Autodesk Inventor part; units mm, degrees
ref_plane "YZ Plane" through (0, 0, 0) normal (1, 0, 0) x (0, 1, 0)
ref_plane "XZ Plane" through (0, 0, 0) normal (0, 1, 0) x (-1, 0, 0)
ref_plane "XY Plane" through (0, 0, 0) normal (0, 0, 1) x (1, 0, 0)
sketch "Sketch1" plane through (0, 0, 0) normal (0, 0, 1) x (1, 0, 0)
  circle A0 centre (10, 11.5) radius 1.6
  line L0 (0, 0) -> (20.0001, 0)
  line L1 (0, 0) -> (0, 3)
  line L2 (20.0001, 0) -> (20.0001, 3)
  line L3 (0, 3) -> (16, 3) construction
  line L4 (20.0001, 3) -> (36.0001, 3) construction
  arc A1 (14.3301, 14) -> (5.6699, 14) centre (10, 11.5) ccw
  line L5 (10, 11.5) -> (5.6699, 14) construction
  line L6 (10, 11.5) -> (14.3301, 14) construction
  line L7 (5.6699, 14) -> (0, 3)
  line L8 (14.3301, 14) -> (20.0001, 3)
  dimension "d17" = 3
  dimension "d18" = 3
  dimension "d19" = 11.5
  dimension "d23" = 90
  dimension "d24" = 90
  dimension "d25" = 10
  dimension "d31" = 5
  dimension "d32" = 120
  dimension "d33" = 14
extrude "Extrusion1" add sketch "Sketch1" along normal blind 4.5
sketch "Sketch4" plane through (0, 0, 4.5) normal (0, 0, 1) x (1, 0, 0)
  line L0 (0, 3) -> (0, 0)
  line L1 (20.0001, 0) -> (20.0001, 3)
  line L2 (0, 0) -> (20.0001, 0)
  line L3 (20.0001, 0) -> (20.0001, 3)
  line L4 (3.884, 22.9404) -> (-0.9789, 3.2417)
  line L5 (20.0001, 3) -> (0, 3)
  line L6 (0, 3) -> (0, 0)
extrude "Extrusion2" add sketch "Sketch4" along normal blind 4.5
sketch "Sketch5" plane through (0, 0, 0) normal (0, -1, 0) x (1, 0, 0)
  circle A0 centre (5, 5) radius 1.6
  circle A1 centre (15, 5) radius 1.6
  line L0 (0, 0) -> (20.0001, 0)
  dimension "d13" = 3.2
  dimension "d14" = 3.2
  dimension "d38" = 5
  dimension "d39" = 5
extrude "Extrusion3" cut sketch "Sketch5" against normal through all
sketch "Sketch6" plane through (0, 3, 9) normal (0, 1, 0) x (1, 0, 0)
  circle A0 centre (5, 4) radius 1.6
  circle A1 centre (5, 4) radius 3
  circle A2 centre (15, 4) radius 1.6
  circle A3 centre (15, 4) radius 3
  line L0 (0, 9) -> (20.0001, 9)
  dimension "d34" = 6
  dimension "d35" = 6
  dimension "d40" = 5
  dimension "d41" = 5
extrude "Extrusion4" cut sketch "Sketch6" along normal up to next
sketch "Sketch7" plane through (0, 0, 0) normal (0, -1, 0) x (1, 0, 0)
  line L0 (0, 0) -> (0, 9)
  line L1 (2.042, 0) -> (0, 0)
  line L2 (0, 0) -> (0, 9)
  line L3 (0, 9) -> (2.042, 9)
  line L4 (2.042, 9) -> (2.042, 0)
extrude "Extrusion5" cut sketch "Sketch7" against normal up to next
sketch "Sketch8" plane through (20.0001, 0, 0) normal (0, -1, 0) x (1, 0, 0)
  line L0 (0, 4.5) -> (0, 9)
  line L1 (-2.042, 0) -> (0, 0)
  line L2 (0, 0) -> (0, 9)
  line L3 (0, 9) -> (-2.042, 9)
  line L4 (-2.042, 9) -> (-2.042, 0)
  point P0 (-20.0001, 0)
extrude "Extrusion6" cut sketch "Sketch8" against normal up to next
properties part number "lower_deck_shaft_mount_for_AD"
Verification items for the finished model (mm, model axes). A direction names the side the tool comes from. Give positions to 0.01 mm unless a question says otherwise; leave off trailing zeros. Loops run counter-clockwise (first coordinate to the right, second up) from the corner with the lowest first, then second, coordinate; pieces in that order, holes last.
1. Section check B-B, the plane z = 4.25. Enter the section's corners in (x, y).
2. Mould release check, pull along Z, two halves, no side actions. Record for faces 1 (the cylindrical face through (14.024, 7.989, 2.163)), 2 (the cylindrical face through (4.65, 1.48, 3.44)), 3 (the flat face through (10, 7, 0)), 4 (the flat face through (17.958, 2.7, 3.6)): released by +Z, released by -Z, zero draft, split by the parting line, or undercut.
3. Set-up check for faces 5 (the flat face through (9.5, 9.8, 4.5)), 6 (the flat face through (10, 3, 6)), 7 (the cylindrical face through (13.4, 1.48, 5.07)): record each of +Z, -Z, +X, -X, +Y, -Y from which the full face is reachable in a straight line by a thin tool's end or side.
4. Thickness scan on line 1 (Z direction, x = 15, y = 1.9); line 2 (Y direction, x = 10, z = 3.15); line 3 (Z direction, x = 11.75, y = 13.5). Record the ranges inside material, lowest first.
5. Section check D-D, the plane y = 11.5. Enter the section's corners in (x, z).
6. Go/stop test with flat-tipped pins: pin 1 Ø1.5 at (x, y) = (5, 11.5) entering from -Z; pin 2 Ø4 at (x, y) = (10, 12) entering from +Z; pin 3 Ø5 at (x, z) = (5, 5) entering from +Y. Record where each tip stops, or that it passes through.
7. Section check A-A, the plane x = 10. Enter the section's corners in (y, z), then the cut area to 4 significant figures.
Geometry says:
1. outline: (2.04, 0) - (3.59, 0) - (3.59, 3) - (2.1, 3) - (2.1, 7.06) - (2.04, 6.96) - close; (6.41, 0) - (13.59, 0) - (13.59, 3) - (12.1, 3) - (12.1, 16.04) arc R5 ccw to (7.9, 16.04) - (7.9, 3) - (6.41, 3) - close; (16.41, 0) - (17.96, 0) - (17.96, 6.96) - (17.9, 7.07) - (17.9, 3) - (16.41, 3) - close; hole circle Ø3.2 at (10, 11.5)
2. face 1: released by +Z
2. face 2: undercut
2. face 3: released by -Z
2. face 4: zero draft
3. face 5: +Z, +X, -X, +Y
3. face 6: +Z, +Y
3. face 7: +Y, -Y
4. line 1: z = 0 to 3.4, 6.6 to 9
4. line 2: y = 0 to 9.9, 13.1 to 16.5
4. line 3: z = 0 to 4.5
5. outline: (4.38, 0) - (8.4, 0) - (8.4, 4.5) - (7.96, 4.5) arc R3 cw to (4.38, 2.06) - close; (11.6, 0) - (15.62, 0) - (15.62, 2.06) arc R3 cw to (12.04, 4.5) - (11.6, 4.5) - close
6. pin 1: stops at z = 0
6. pin 2: stops at z = 4.5
6. pin 3: stops at y = 3
7. outline: (0, 0) - (9.9, 0) - (9.9, 4.5) - (3, 4.5) - (3, 9) - (0, 9) - close; (13.1, 0) - (16.5, 0) - (16.5, 4.5) - (13.1, 4.5) - close
7. area: 73.35 mm2
